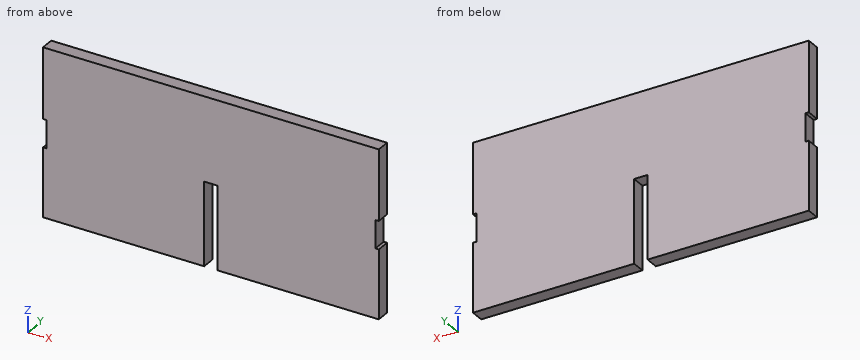
```python
from build123d import *

# Parameters (mm, degrees)
F0_W     = 6
F0_H     = 50
F1_DEPTH = 24
F2_DEPTH = 96


with BuildPart() as f1:
    # F0 (on Front) → F1 (new body)
    with BuildSketch(Plane.XZ):
        Polygon((230.500006, 138), (-369.499994, 138), (-369.499994, 12), (-363.499994, 12), (-363.499994, -38), (-369.499994, -38), (-369.499994, -161), (-81.499994, -161), (-81.499994, -12), (-57.499994, -12), (-57.499994, -161), (230.500006, -161), (230.500006, -38), (224.500006, -38), (224.500006, 12), (230.500006, 12), align=None)
        with Locations((-366.499994, -13)):
            Rectangle(F0_W, F0_H)
        with Locations((227.500006, -13)):
            Rectangle(F0_W, F0_H)
    extrude(amount=F1_DEPTH)

    # F0 (on Front) → F2 (cut)
    with BuildSketch(Plane.XZ):
        with Locations((-366.499994, -13)):
            Rectangle(F0_W, F0_H)
        with Locations((227.500006, -13)):
            Rectangle(F0_W, F0_H)
    extrude(amount=F2_DEPTH, mode=Mode.SUBTRACT)


solid = f1.part
```
Input: part model. Units: mm. Frame: model coordinates. Coordinates: 2 decimals unless noted, no trailing zeros. Write each loop counter-clockwise with the first axis right and the second up, starting at its lowest first coordinate (ties: lowest second). Pieces come first, ordered by that corner, then holes.
1) Material intervals for line 1 along X through (y, z) = (-12.25, -56); line 2 along Z through (x, y) = (-79.5, -11), sorted ascending.
2) Section A-A on z = -114.5. Output: boundary loops of the cut face in (x, y), and give its area (3 significant figures).
3) Section B-B on y = -8.5. Output: boundary loops of the cut face in (x, z).
4) Pin query (flat end, axial travel): pin 1 Ø12 at (y, z) = (-15.5, -12.5) entering from +X. Return the tip coordinate at first contact, or that it passes through.
Check result:
1. line 1: x = -369.5 to -81.5, -57.5 to 230.5
1. line 2: z = -12 to 138
2. outline: (-369.5, -24) - (-81.5, -24) - (-81.5, 0) - (-369.5, 0) - close; (-57.5, -24) - (230.5, -24) - (230.5, 0) - (-57.5, 0) - close
2. area: 13,800 mm2
3. outline: (-369.5, -161) - (-81.5, -161) - (-81.5, -12) - (-57.5, -12) - (-57.5, -161) - (230.5, -161) - (230.5, -38) - (224.5, -38) - (224.5, 12) - (230.5, 12) - (230.5, 138) - (-369.5, 138) - (-369.5, 12) - (-363.5, 12) - (-363.5, -38) - (-369.5, -38) - close
4. pin 1: stops at x = 224.5
